from build123d import *

# Parameters (mm, degrees)
LINEAR_AUSTRAGEN_D_NN1_DEPTH      = 2
LINEAR_AUSTRAGEN_D_NN1_DEPTH_BACK = 2


with BuildPart() as part:
    # Skizze1 → Linear-Austragen-D_nn1 (new body, two sides)
    with BuildSketch(Plane(origin=(0, 0, 0), x_dir=(1, 0, 0), z_dir=(0, 1, 0))) as linear_austragen_d_nn1_sk:
        with BuildLine():
            Line((40.65321754, -14.567567699), (-1.169276765, -5.246276474))
            ThreePointArc((-1.169276765, -5.246276474), (-5.375, 0), (-1.169276765, 5.246276474))
            Line((-1.169276765, 5.246276474), (40.65321754, 14.567567699))
            ThreePointArc((40.65321754, 14.567567699), (58.825, 0), (40.65321754, -14.567567699))
        make_face()
        with BuildLine():
            Line((40.827249431, -13.786726549), (-0.995244875, -4.465435325))
            ThreePointArc((-0.995244875, -4.465435325), (-4.575, 0), (-0.995244875, 4.465435325))
            Line((-0.995244875, 4.465435325), (40.827249431, 13.786726549))
            ThreePointArc((40.827249431, 13.786726549), (58.025, 0), (40.827249431, -13.786726549))
        make_face(mode=Mode.SUBTRACT)
    extrude(amount=LINEAR_AUSTRAGEN_D_NN1_DEPTH)
    extrude(linear_austragen_d_nn1_sk.sketch, amount=-LINEAR_AUSTRAGEN_D_NN1_DEPTH_BACK)


solid = part.part
Input: part model. Units: mm. Frame: model coordinates. A direction names the side the tool comes from. Coordinates: 2 decimals unless noted, no trailing zeros. Loops run counter-clockwise (first coordinate to the right, second up) from the corner with the lowest first, then second, coordinate; pieces in that order, holes last. Notation, with made-up numbers: (64, -18) -> (81, -18) arc R26 cw to (81, 10) -> close; hole circle Ø2 at (65, -7). An arc over 180 degrees is marked (long way). Write each question's results on one line, items separated by ' | '. Start each with the question number.
Q1. Section C-C, the plane y = -0.8. Return the cut outline in (x, z) (3 decimals), plus the area to 3 significant figures.
Q2. Section A-A, the plane z = 0. Return the cut outline in (x, y) (3 decimals).
Q3. Ray query, line 1 (Z direction, x = 43.9, y = -0.85) (3 decimals); line 2 (X direction, y = -1.1, z = 0) (3 decimals); line 3 (Z direction, x = 40, y = 0.2). Return the intervals inside material, ascending. Write a range as from..to.
Q4. Section B-B, the plane x = 44. Return the cut outline in (y, z), plus the area to 3 significant figures.
Q5. Pin query (flat end, axial travel): pin 1 (1.5 mm diameter, centred on x = 9, y = 1, fed in from +Z); pin 2 (2 mm diameter, centred on x = 33, y = -0.5, fed in from -Z); pin 3 (1.5 mm diameter, centred on x = 2, y = -1, fed in from -Z). Return the tip coordinate at first contact, or that it passes through.
Q6. Reachability of faces 1 (the flat face through (19.45, 0.03, -9.84)), 2 (the cylindrical face through (-4.574, 0.028, 0.087)) from +Z, -Z, +X, -X, +Y, -Y: full face, straight path, thin tool, end or side. Return the list, or none.
Q7. Pull-direction query (X, two-part tool) for faces 3 (the flat face through (27, -2, 11)), 4 (the flat face through (20.21, 0.03, 9.19)), 5 (the flat face through (19.62, 0.03, -9.06)), 6 (the flat face through (20.03, 0.03, 9.97)); classes: released by +X, released by -X, zero draft, split by the parting line, or undercut.
Found:
1) outline: (-1.169, -5.246) -> (40.653, -14.568) arc R14.925 ccw (long way) to (40.653, 14.568) -> (-1.169, 5.246) arc R5.375 ccw to start; hole (-0.995, -4.465) -> (40.827, -13.787) arc R14.125 ccw (long way) to (40.827, 13.787) -> (-0.995, 4.465) arc R4.575 ccw to start | area: 121 mm2
2) outline: (-5.375, -2) -> (-4.575, -2) -> (-4.575, 2) -> (-5.375, 2) -> close; (58.025, -2) -> (58.825, -2) -> (58.825, 2) -> (58.025, 2) -> close
3) line 1: -14.925..-14.125, 14.125..14.925 | line 2: -5.375..-4.575, 58.025..58.825 | line 3: -14.42..-13.6, 13.6..14.42
4) outline: (-2, -14.92) -> (2, -14.92) -> (2, -14.12) -> (-2, -14.12) -> close; (-2, 14.12) -> (2, 14.12) -> (2, 14.92) -> (-2, 14.92) -> close | area: 6.40 mm2
5) pin 1: z = 7.68 | pin 2: z = -13.08 | pin 3: z = -6.12
6) face 1: -Z, -X, +Y, -Y | face 2: +Y, -Y
7) face 3: zero draft | face 4: undercut | face 5: undercut | face 6: released by -X
